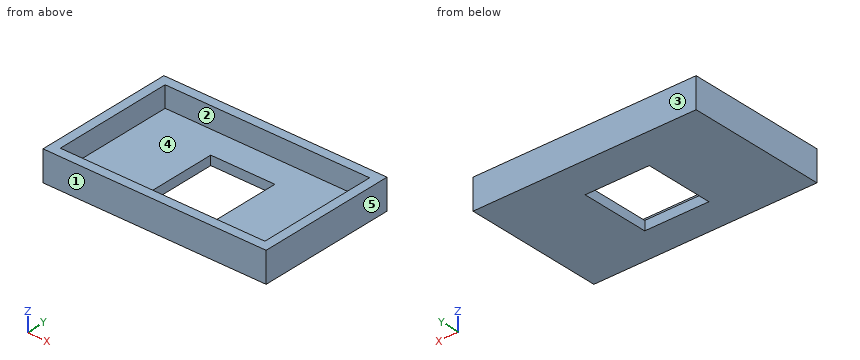
```python
from build123d import *

# Parameters (mm, degrees)
SKETCH_W      = 48
SKETCH_H      = 30
PAD_DEPTH     = 2
SKETCH001_W   = 48
SKETCH001_H   = 30
SKETCH001_W_2 = 44
SKETCH001_H_2 = 26
PAD001_DEPTH  = 4.5
SKETCH002_W   = 13.8
SKETCH002_H   = 14.8
POCKET_DEPTH  = 2


with BuildPart() as part:
    # Sketch → Pad (new body)
    with BuildSketch(Plane.XY):
        with Locations((24, 15)):
            Rectangle(SKETCH_W, SKETCH_H)
    extrude(amount=PAD_DEPTH)

    # Sketch001 (on Face6 of Pad) → Pad001 (join)
    with BuildSketch(Plane.XY.offset(2)):
        with Locations((24, 15)):
            Rectangle(SKETCH001_W, SKETCH001_H)
        with Locations((24, 15)):
            Rectangle(SKETCH001_W_2, SKETCH001_H_2, mode=Mode.SUBTRACT)
    extrude(amount=PAD001_DEPTH)

    # Sketch002 (on Face15 of Pad001) → Pocket (cut)
    with BuildSketch(Plane.XY.offset(2)):
        with Locations((24, 14.5)):
            Rectangle(SKETCH002_W, SKETCH002_H)
    extrude(amount=-POCKET_DEPTH, mode=Mode.SUBTRACT)


solid = part.part
```
Input: part model. Units: mm. Frame: model coordinates. Face numbers are marked on the shaded views. A direction names the side the tool comes from. Coordinates: 2 decimals unless noted, no trailing zeros. Write each loop counter-clockwise with the first axis right and the second up, starting at its lowest first coordinate (ties: lowest second). Pieces come first, ordered by that corner, then holes. Notation, with made-up numbers: M -7,-26 L 13,-26 A25 ccw 13,-14 Z; hole C 41,79 d9. An arc over 180 degrees is marked long. Use one line per item in the form item = value.
Q1. First-contact query: pin 1 (8 mm diameter, centred on x = 30.5, y = 18.5, fed in from +Z). Flat tip, straight axial feed; report the tip coordinate or a pass-through.
Answer below:
pin_1 = 2
Q2. Section B-B (y = 17). Return loops of the section in (x, z).
Answer below:
outline = M 0,0 L 17.1,0 L 17.1,2 L 2,2 L 2,6.5 L 0,6.5 Z; M 30.9,0 L 48,0 L 48,6.5 L 46,6.5 L 46,2 L 30.9,2 Z
Q3. Set-up query: the marked faces 1 and 2. Return all of +Z, -Z, +X, -X, +Y, -Y with unobstructed straight access to the full face (end or side cutting, diameter ignored); none if empty.
Answer below:
face_1 = +Z, -Z, +X, -X, -Y
face_2 = +Z
Q4. Section C-C (z = 4.75). Return loops of the section in (x, y), plus the area to 3 significant figures.
Answer below:
outline = M 0,0 L 48,0 L 48,30 L 0,30 Z; hole M 2,2 L 46,2 L 46,28 L 2,28 Z
area = 296 mm²
Q5. Section D-D (x = 5). Return loops of the section in (y, z).
Answer below:
outline = M 0,0 L 30,0 L 30,6.5 L 28,6.5 L 28,2 L 2,2 L 2,6.5 L 0,6.5 Z
Q6. Material intervals for probe 1 along X at (y, z) = (19, 3); probe 2 along Y at (x, z) = (15, 2.5); probe 3 along X at (y, z) = (8.5, 1.75), sorted ascending. Write a range as from..to.
Answer below:
probe_1 = 0..2, 46..48
probe_2 = 0..2, 28..30
probe_3 = 0..17.1, 30.9..48
Q7. Section A-A (x = 29). Return loops of the section in (y, z).
Answer below:
outline = M 0,0 L 7.1,0 L 7.1,2 L 2,2 L 2,6.5 L 0,6.5 Z; M 21.9,0 L 30,0 L 30,6.5 L 28,6.5 L 28,2 L 21.9,2 Z
Q8. Draft query along Y for the marked faces 3, 4 and 5. Return one class per face: released by +Y, released by -Y, zero draft, split by the parting line, or undercut.
Answer below:
face_3 = released by +Y
face_4 = undercut
face_5 = zero draft
